```python
from build123d import *

# Parameters (mm, degrees)
SKETCH_2_W         = 28.5
SKETCH_2_H         = 16
SKETCH_2_R         = 1.5
EXTRUDE_1_DEPTH    = 3
HOLE_WIZARD_M3_2_D = 2.5
CHAMFER_1_SIZE     = 0.5


with BuildPart() as part:
    # 草图2 → 凸台-拉伸1 (new body, symmetric)
    with BuildSketch(Plane.XY):
        with Locations((-11.25, 0)):
            Rectangle(SKETCH_2_W, SKETCH_2_H)
        with Locations((-15, 0)):
            Circle(SKETCH_2_R, mode=Mode.SUBTRACT)
        Circle(SKETCH_2_R, mode=Mode.SUBTRACT)
    extrude(amount=EXTRUDE_1_DEPTH, both=True)

    # M3 螺纹孔2 (through all)
    with Locations(Plane(origin=(0, 8, 0), x_dir=(1, 0, 0), z_dir=(0, 1, 0))):
        with Locations((-7.5, 0), (-22.5, 0)):
            Hole(HOLE_WIZARD_M3_2_D / 2)

    # 倒角1
    chamfer_1_edges = [part.edges().sort_by_distance(p)[0] for p in [
        (-11.25, -8, 3),
        (3, 0, 3),
        (-11.25, 8, 3),
        (3, 0, -3),
        (-11.25, -8, -3),
        (-25.5, 0, -3),
        (-11.25, 8, -3),
        (-25.5, 0, 3),
        (3, 8, 0),
        (3, -8, 0),
        (-25.5, -8, 0),
        (-25.5, 8, 0),
    ]]
    chamfer(chamfer_1_edges, length=CHAMFER_1_SIZE)


solid = part.part
```
Check sheet for the modelled part. Datum: model origin and axes. Units: mm. Give positions to 0.01 mm unless a question says otherwise; leave off trailing zeros. Loops run counter-clockwise (first coordinate to the right, second up) from the corner with the lowest first, then second, coordinate; pieces in that order, holes last. Notation, with made-up numbers: M 84.5,73.25 L 130.5,73.25 A22 ccw 130.5,79.25 Z; hole C -8,9.25 d10. An arc over 180 degrees is marked long. Answer in a Markdown table with one row per item.
1) Cross-section at C-C (y = 0). Enter the section's corners in (x, z), plus the area to 3 significant figures.
Solutions:
| item | result |
|---|---|
| outline | M -25.5,-2.5 L -25,-3 L -16.5,-3 L -16.5,3 L -25,3 L -25.5,2.5 Z; M -13.5,-3 L -1.5,-3 L -1.5,3 L -13.5,3 Z; M 1.5,-3 L 2.5,-3 L 3,-2.5 L 3,2.5 L 2.5,3 L 1.5,3 Z; hole C -22.5,0 d2.5; hole C -7.5,0 d2.5 |
| area | 125 mm^2 |
2) Mould release check, pull along X, two halves, no side actions. Record for faces 1 (the face through (3, 0, 0)), 2 (the face through (-16.5, 0.07, -0.04)), 3 (the face through (-11, 0, -3)): released by +X, released by -X, zero draft, split by the parting line, or undercut.
Solutions:
| item | result |
|---|---|
| face 1 | released by +X |
| face 2 | undercut |
| face 3 | zero draft |
3) Cross-section at B-B (x = -7.5). Enter the section's corners in (y, z), plus the area to 3 significant figures.
Solutions:
| item | result |
|---|---|
| outline | M -8,-2.5 L -7.5,-3 L 7.5,-3 L 8,-2.5 L 8,-1.25 L -8,-1.25 Z; M -8,1.25 L 8,1.25 L 8,2.5 L 7.5,3 L -7.5,3 L -8,2.5 Z |
| area | 55.5 mm^2 |
4) Cross-section at D-D (y = 6.75). Enter the section's corners in (x, z), plus the area to 3 significant figures.
Solutions:
| item | result |
|---|---|
| outline | M -25.5,-2.5 L -25,-3 L 2.5,-3 L 3,-2.5 L 3,2.5 L 2.5,3 L -25,3 L -25.5,2.5 Z; hole C -22.5,0 d2.5; hole C -7.5,0 d2.5 |
| area | 161 mm^2 |
5) Thickness scan on line 1 (Z direction, x = -22.5, y = 1.25); line 2 (X direction, y = 0.75, z = 2.25); line 3 (X direction, y = 0.25, z = 1). Record the ranges inside material, lowest first.
Solutions:
| item | result |
|---|---|
| line 1 | z = -3 to -1.25, 1.25 to 3 |
| line 2 | x = -25.5 to -16.3, -13.7 to -1.3, 1.3 to 3 |
| line 3 | x = -25.5 to -23.25, -21.75 to -16.48, -13.52 to -8.25, -6.75 to -1.48, 1.48 to 3 |
6) Cross-section at A-A (z = 0). Enter the section's corners in (x, y), plus the area to 3 significant figures.
Solutions:
| item | result |
|---|---|
| outline | M -25.5,-7.5 L -25,-8 L -23.75,-8 L -23.75,8 L -25,8 L -25.5,7.5 Z; M -21.25,-8 L -8.75,-8 L -8.75,8 L -21.25,8 Z; M -6.25,-8 L 2.5,-8 L 3,-7.5 L 3,7.5 L 2.5,8 L -6.25,8 Z; hole C -15,0 d3; hole C 0,0 d3 |
| area | 361 mm^2 |
